Input: dimensioned drawing with shaded views. Units: mm. Origin: part minimum x, y, z. A direction names the side the tool comes from. Give positions to 0.01 mm unless a question says otherwise; leave off trailing zeros. Loops run counter-clockwise (first coordinate to the right, second up) from the corner with the lowest first, then second, coordinate; pieces in that order, holes last. Notation, with made-up numbers: (2, 81) -> (31, 81) arc R35 cw to (31, 120) -> close; hole circle Ø6 at (65.25, -12.75). An arc over 180 degrees is marked (long way). Answer in a Markdown table with one row per item. Add a question column.
1) Access query for the marked faces 4 and 5. Directions: +Z, -Z, +X, -X, +Y, -Y. A direction counts if a zero-diameter tool reaches every point of the face in a straight line with its end or side. Return the directions, or none.
2) First-contact query: P1, Ø9, axis at y = 47.5, z = 47.5, coming from the -X side; P2, Ø12, axis at x = 12.5, y = 10, coming from the -Z side; P3, Ø10, axis at x = 44, y = 59.5, coming from the +Z side; P4, Ø10, axis at x = 32, z = 57.5, coming from the -Y side. Flat tips, straight axial feed; report the tip coordinate or a pass-through.
3) Section query B-B (x = 52). Return the cut outline in (y, z).
4) Section query A-A (z = 47.5). Return the cut outline in (x, y), plus the area to 3 significant figures.
5) Draft query along Y for the marked faces 1, 2 and 3. Return one class per face: +Y half, -Y half, draft (parallel to the pull), parting line (faces both ways), or undercut.
6) Section query C-C (x = 19.5). Return the cut outline in (y, z), plus the area to 3 significant figures.
7) Line query: line 1 (X direction, y = 67, z = 58.5); line 2 (X direction, y = 63, z = 69); line 3 (Y direction, x = 53, z = 47). Output: solid intervals per line, ascending. Write a range as from..to.
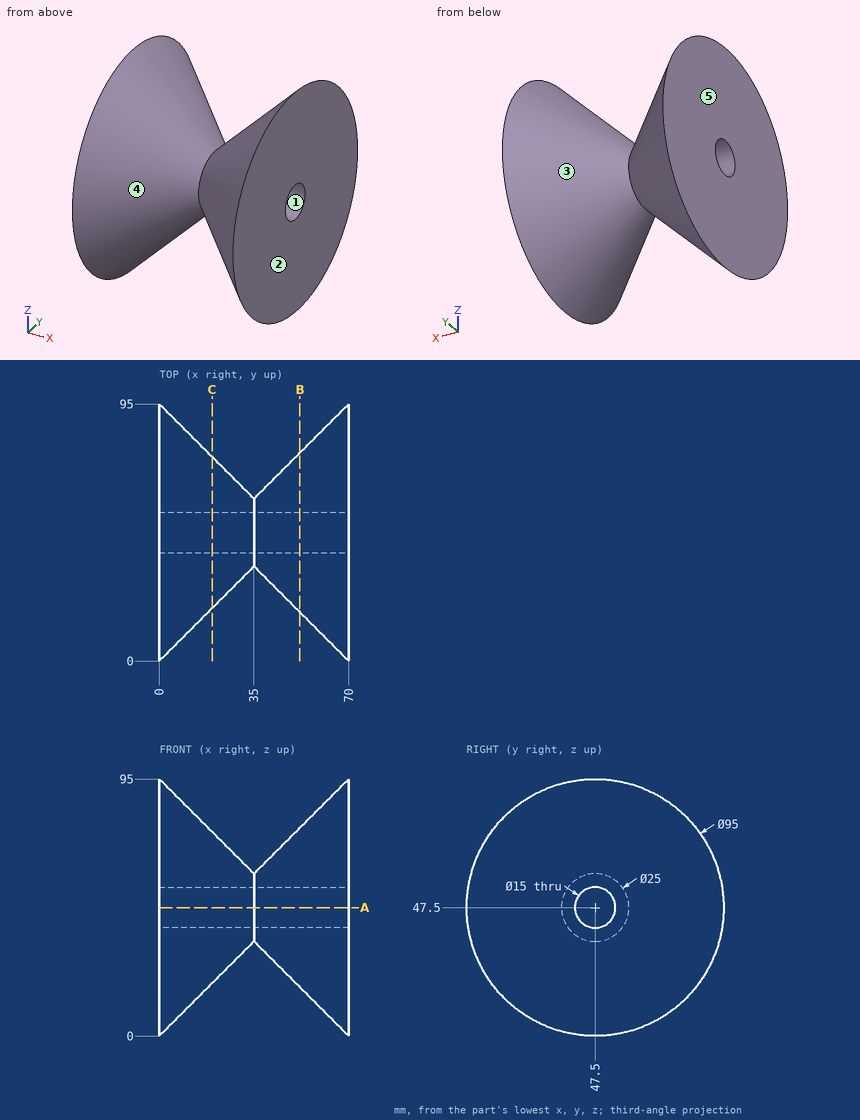
Evaluation:
| question | item | result |
|---|---|---|
| 1 | face 4 | none |
| 1 | face 5 | +Z, -Z, -X, +Y, -Y |
| 2 | P1 | through |
| 2 | P2 | z = 26.62 |
| 2 | P3 | z = 71.59 |
| 2 | P4 | y = 29.08 |
| 3 | outline | circle Ø59 at (47.5, 47.5); hole circle Ø15 at (47.5, 47.5) |
| 4 | outline | (0, 0) -> (35, 35) -> (70, 0) -> (70, 40) -> (0, 40) -> close; (0, 55) -> (70, 55) -> (70, 95) -> (35, 60) -> (0, 95) -> close |
| 4 | area | 3,150 mm² |
| 5 | face 1 | undercut |
| 5 | face 2 | draft |
| 5 | face 3 | parting line |
| 6 | outline | circle Ø56 at (47.5, 47.5); hole circle Ø15 at (47.5, 47.5) |
| 6 | area | 2,290 mm² |
| 7 | line 1 | 0..25.11, 44.89..70 |
| 7 | line 2 | 0..21, 49..70 |
| 7 | line 3 | 17..40.02, 54.98..78 |
